Part model, mm, in its own coordinate system. A direction names the side the tool comes from. Coordinates: 2 decimals unless noted, no trailing zeros. Write each loop counter-clockwise with the first axis right and the second up, starting at its lowest first coordinate (ties: lowest second). Pieces come first, ordered by that corner, then holes. Notation, with made-up numbers: (2, -1) -> (52, -1) arc R22 ccw to (52, 22) -> close; hole circle Ø10 at (43.5, 39.25). An arc over 180 degrees is marked (long way). Write item = value, one per line. Start each with the question number.
Q1. Pull direction X, two halves, no side cores. Call faces 5 (the flat face through (38.1, 0, 6)), 6 (the flat face through (-28, 0, 0)), 7 (the cylindrical face through (7.956, -7.296, 28.619)): released by +X, released by -X, zero draft, split by the parting line, or undercut.
Q2. Band-saw the part on A-A, the plane z = 8. List the corners of the cut face in (x, y) (3 decimals), plus the area to 3 significant figures.
Q3. Tool access for faces 1 (the cylindrical face through (15.12, 11.59, 22.09)), 2 (the cylindrical face through (1.82, -13.85, 22.27)), 3 (the flat face through (-27, 0, 12.7)), 4 (the flat face through (27, 0, 0)): list every direction of +Z, -Z, +X, -X, +Y, -Y with a clear straight run to the whole face (end or side of a thin tool).
Q4. Probe line 1 (Z direction, x = 10.5, y = 8.5); line 2 (X direction, y = 0, z = 9) (3 decimals); line 3 (X direction, y = 0, z = 20). List the from-to ranges inside material, lowest first.
Q5. Band-saw the part on B-B, the plane x = -9.5. List the corners of the cut face in (y, z).
Q6. Band-saw the part on C-C, the plane y = 12. List the corners of the cut face in (x, z).
Q7. Band-saw the part on D-D, the plane y = 3.5. List the corners of the cut face in (x, z), plus the area to 3 significant figures.
Q8. Pin check, flat tips, straight feed: P1, Ø5, axis at x = 14, z = -3, coming from the +Y side; P2, Ø8, axis at x = -19, z = -12.5, coming from the +Y side; P3, Ø4, axis at y = 12, z = 21, coming from the -X side; P4, Ø8, axis at x = 1, z = 23, coming from the -Y side. Stop position of each tip, or through.
from build123d import *

# Parameters (mm, degrees)
F1_DEPTH  = 19.05
F3_FACE_R = 10.795
F4_DEPTH  = 25.4
F5_R      = 10.795
F6_DEPTH  = 19.05


with BuildPart() as f1:
    # F0 (on Front) → F1 (new body, symmetric)
    with BuildSketch(Plane.XZ):
        Polygon((-38.1, 0), (0, 0), (38.1, 0), (38.1, 12.7), (-38.1, 12.7), align=None)
    extrude(amount=F1_DEPTH, both=True)

    # F2 (on Front) → F3 (revolve)
    with BuildSketch(Plane.XZ):
        Polygon((-19.05, 31.75), (-19.05, 12.7), (-10.795, 12.7), (-10.795, 19.05), (-13.97, 19.05), (-13.97, 25.4), (-10.795, 25.4), (-10.795, 31.75), align=None)
    revolve(axis=Axis((0, 0, 15.662436), (0, 0, 1)))

    # F3_face (on face) → F4 (cut)
    with BuildSketch(Plane.XY.offset(12.7)):
        Circle(F3_FACE_R)
    extrude(amount=-F4_DEPTH, mode=Mode.SUBTRACT)

    # F5 (on face) → F6 (join)
    with BuildSketch(Plane(origin=(0, 0, 0), x_dir=(1, 0, 0), z_dir=(0, 0, -1))):
        with BuildLine():
            ThreePointArc((0, -19.05), (13.470384, -13.470384), (19.05, 0))
            ThreePointArc((19.05, 0), (13.470384, 13.470384), (0, 19.05))
            ThreePointArc((0, 19.05), (-19.05, 0), (0, -19.05))
        make_face()
        Circle(F5_R, mode=Mode.SUBTRACT)
    extrude(amount=F6_DEPTH)


solid = f1.part
Ans:
q1.face_5 = released by +X
q1.face_6 = zero draft
q1.face_7 = undercut
q2.outline = (-38.1, -19.05) -> (38.1, -19.05) -> (38.1, 19.05) -> (-38.1, 19.05) -> close; hole circle Ø21.59 at (0, 0)
q2.area = 2,540 mm2
q3.face_1 = +Z
q3.face_2 = none
q3.face_3 = +Z, -X
q3.face_4 = -Z, +X
q4.line_1 = -19.05 to 19.05, 25.4 to 31.75
q4.line_2 = -38.1 to -10.795, 10.795 to 38.1
q4.line_3 = -19.05 to -13.97, 13.97 to 19.05
q5.outline = (-19.05, 0) -> (-16.51, 0) -> (-16.51, -19.05) -> (-5.13, -19.05) -> (-5.13, 19.05) -> (-10.24, 19.05) -> (-10.24, 25.4) -> (-5.13, 25.4) -> (-5.13, 31.75) -> (-16.51, 31.75) -> (-16.51, 12.7) -> (-19.05, 12.7) -> close; (5.13, -19.05) -> (16.51, -19.05) -> (16.51, 0) -> (19.05, 0) -> (19.05, 12.7) -> (16.51, 12.7) -> (16.51, 31.75) -> (5.13, 31.75) -> (5.13, 25.4) -> (10.24, 25.4) -> (10.24, 19.05) -> (5.13, 19.05) -> close
q6.outline = (-38.1, 0) -> (-14.8, 0) -> (-14.8, -19.05) -> (14.8, -19.05) -> (14.8, 0) -> (38.1, 0) -> (38.1, 12.7) -> (14.8, 12.7) -> (14.8, 31.75) -> (-14.8, 31.75) -> (-14.8, 12.7) -> (-38.1, 12.7) -> close; hole (-7.15, 19.05) -> (7.15, 19.05) -> (7.15, 25.4) -> (-7.15, 25.4) -> close
q7.outline = (-38.1, 0) -> (-18.73, 0) -> (-18.73, -19.05) -> (-10.21, -19.05) -> (-10.21, 19.05) -> (-13.52, 19.05) -> (-13.52, 25.4) -> (-10.21, 25.4) -> (-10.21, 31.75) -> (-18.73, 31.75) -> (-18.73, 12.7) -> (-38.1, 12.7) -> close; (10.21, -19.05) -> (18.73, -19.05) -> (18.73, 0) -> (38.1, 0) -> (38.1, 12.7) -> (18.73, 12.7) -> (18.73, 31.75) -> (10.21, 31.75) -> (10.21, 25.4) -> (13.52, 25.4) -> (13.52, 19.05) -> (10.21, 19.05) -> close
q7.area = 1,320 mm2
q8.P1 = 15.19
q8.P2 = 11.74
q8.P3 = -16.21
q8.P4 = -19.05
